Could you check a few things on this model? Use its own coordinates, in mm. Face numbers are marked on the shaded views. A direction names the side the tool comes from. Coordinates: 2 decimals unless noted, no trailing zeros. Write each loop counter-clockwise with the first axis right and the second up, starting at its lowest first coordinate (ties: lowest second). Pieces come first, ordered by that corner, then holes. Notation, with made-up numbers: M 31,-4.5 L 38,-4.5 A16 ccw 38,12.5 Z; hole C 18.5,73.5 d10. An arc over 180 degrees is marked long. Write item = value, one per line.
```python
from build123d import *

# Parameters (mm, degrees)
SKETCH083_R     = 16
SKETCH083_R_2   = 6
PAD029_DEPTH    = 7.95
SKETCH084_R     = 13.5
SKETCH084_R_2   = 7.75
POCKET048_DEPTH = 1


with BuildPart() as part:
    # Sketch083 → Pad029 (new body, symmetric)
    with BuildSketch(Plane.XY):
        Circle(SKETCH083_R)
        Circle(SKETCH083_R_2, mode=Mode.SUBTRACT)
    extrude(amount=PAD029_DEPTH, both=True)

    # Sketch084 (on Face4 of Pad029) → Pocket048 (cut)
    with BuildSketch(Plane.XY.offset(7.95)):
        Circle(SKETCH084_R)
        Circle(SKETCH084_R_2, mode=Mode.SUBTRACT)
    pocket048 = extrude(amount=-POCKET048_DEPTH, mode=Mode.SUBTRACT)

    # Mirrored001: Pocket048 across XY
    add(pocket048.mirror(Plane.XY), mode=Mode.SUBTRACT)


solid = part.part
```
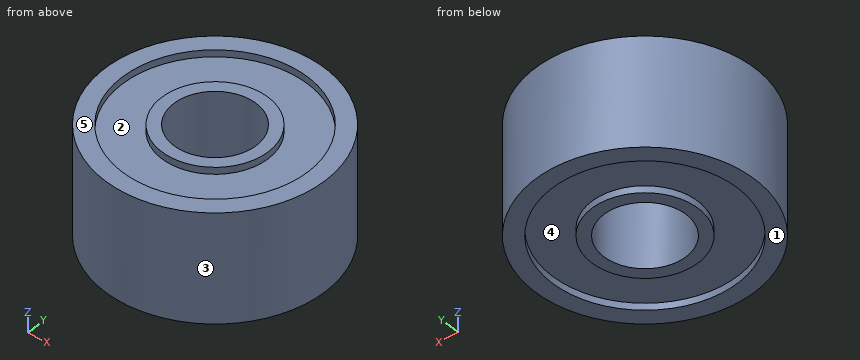
Item 1: I'm going to push flat-ended pins straight in: P1, Ø3, axis at x = -5, z = 6, coming from the -Y side; P2, Ø6, axis at y = -1.5, z = 5.5, coming from the -X side; P3, Ø5, axis at y = 7.5, z = -5.5, coming from the +X side; P4, Ø1, axis at x = -2.5, z = 3.5, coming from the +Y side. Where does each tip first touch, or does it pass through?
Numbers:
P1 = -15.61
P2 = -16
P3 = 15.2
P4 = 15.87
Item 2: Imagine slicing it at D-D (x = -14). Write out the boundary of the cut face in (y, z), and give its area (3 significant figures).
Numbers:
outline = M -7.75,-7.95 L 7.75,-7.95 L 7.75,7.95 L -7.75,7.95 Z
area = 246 mm²
Item 3: For the marked faces 4 and 5, which set-ups out of +Z, -Z, +X, -X, +Y, -Y let a thin tool reach every point of the face, with its end or its side?
Numbers:
face_4 = -Z
face_5 = +Z, +X, -X, +Y, -Y
Item 4: Imagine slicing it at C-C (z = -1.25). Write out the boundary of the cut face in (x, y), and give its area (3 significant figures).
Numbers:
outline = C 0,0 d32; hole C 0,0 d12
area = 691 mm²
Item 5: If we mould it in two halves opening along Y, with no side actions, what happens to the marked faces 1, 2 and 3? For each: pulls with the +Y half, pulls with the -Y half, needs draft (parallel to the pull), parting line crosses it, or undercut.
Numbers:
face_1 = needs draft
face_2 = undercut
face_3 = parting line crosses it
Item 6: Imagine slicing it at A-A (x = 0). Write out the boundary of the cut face in (y, z).
Numbers:
outline = M -16,-7.95 L -13.5,-7.95 L -13.5,-6.95 L -7.75,-6.95 L -7.75,-7.95 L -6,-7.95 L -6,7.95 L -7.75,7.95 L -7.75,6.95 L -13.5,6.95 L -13.5,7.95 L -16,7.95 Z; M 6,-7.95 L 7.75,-7.95 L 7.75,-6.95 L 13.5,-6.95 L 13.5,-7.95 L 16,-7.95 L 16,7.95 L 13.5,7.95 L 13.5,6.95 L 7.75,6.95 L 7.75,7.95 L 6,7.95 Z
Item 7: If I drill on line 1 along Y through (x, z) = (0, 7.25); line 2 along Y through (x, z) = (0, -2); line 3 along Z through (x, y) = (-7, -5), over which ranges is the centre line in solid material (lowest first)?
Numbers:
line_1 = -16 to -13.5, -7.75 to -6, 6 to 7.75, 13.5 to 16
line_2 = -16 to -6, 6 to 16
line_3 = -6.95 to 6.95
